from build123d import *

# Parameters (mm, degrees)
SKETCH1_W               = 15
SKETCH1_H               = 15
SKETCH1_R               = 2.5
BOSS_EXTRUDE1_DEPTH     = 90
SKETCH2_W               = 10.174
SKETCH2_H               = 10.174
CUT_EXTRUDE1_DEPTH      = 83
CUT_EXTRUDE2_DEPTH      = 83
CUT_EXTRUDE2_DEPTH_BACK = 83
SKETCH4_R               = 1.75
CUT_EXTRUDE3_DEPTH      = 83


with BuildPart() as part:
    # Sketch1 → Boss-Extrude1 (new body)
    with BuildSketch(Plane(origin=(0, 0, 0), x_dir=(1, 0, 0), z_dir=(0, 1, 0))):
        Rectangle(SKETCH1_W, SKETCH1_H)
        with Locations(Location((0, 0, 0), (0, 0, 270))):
            Circle(SKETCH1_R, mode=Mode.SUBTRACT)
    extrude(amount=-BOSS_EXTRUDE1_DEPTH)

    # Sketch2 → Cut-Extrude1 (cut)
    with BuildSketch(Plane(origin=(0, 0, 0), x_dir=(1, 0, 0), z_dir=(0, 1, 0))):
        Rectangle(SKETCH2_W, SKETCH2_H)
    extrude(amount=-CUT_EXTRUDE1_DEPTH, mode=Mode.SUBTRACT)

    # Sketch3 → Cut-Extrude2 (cut, two sides: drawn at the far end of the back side and taken through both)
    with BuildSketch(Plane(origin=(0, 0, 0), x_dir=(0, 0, -1), z_dir=(1, 0, 0)).offset(-CUT_EXTRUDE2_DEPTH_BACK)):
        Polygon((-7.5, 0), (7.5, -15), (7.5, 0), align=None)
    extrude(amount=CUT_EXTRUDE2_DEPTH + CUT_EXTRUDE2_DEPTH_BACK, mode=Mode.SUBTRACT)

    # Sketch4 → Cut-Extrude3 (cut)
    with BuildSketch(Plane.XY):
        with Locations((0, -10)):
            Circle(SKETCH4_R)
        with Locations((0, -20)):
            Circle(SKETCH4_R)
    extrude(amount=CUT_EXTRUDE3_DEPTH, mode=Mode.SUBTRACT)


solid = part.part
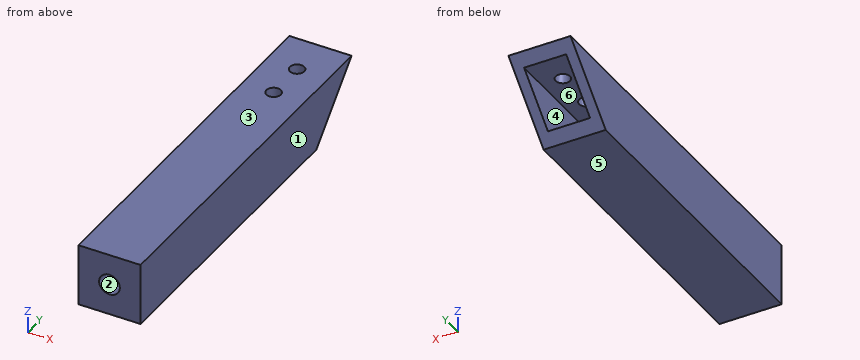
Source: CAD feature listing. Evaluate the final solid. Frame: model axes, mm. Face numbers are marked on the shaded views. A direction names the side the tool comes from. Round coordinates to 2 decimals unless told otherwise and drop trailing zeros. Loops run counter-clockwise (first coordinate to the right, second up) from the corner with the lowest first, then second, coordinate; pieces in that order, holes last. Notation, with made-up numbers: (54, 86.5) - (98, 86.5) arc R29 ccw to (98, 125.5) - close; hole circle Ø2 at (39.25, 21.5). An arc over 180 degrees is marked (long way). Write item = value, one per line. Start each with the question number.
Item 1: Section query A-A on z = 0. Output: boundary loops of the cut face in (x, y), plus the area to 3 significant figures.
Item 2: Mould query, pull axis Z, two halves, no side actions, for the marked faces 1, 2, 3 and 4. Classes: released by +Z, released by -Z, zero draft, split by the parting line, or undercut.
Item 3: Reachability of the marked faces 5 and 6 from +Z, -Z, +X, -X, +Y, -Y: full face, straight path, thin tool, end or side. Return the list, or none.
Item 4: First-contact query: pin 1 Ø5 at (x, z) = (2, -2) entering from +Y; pin 2 Ø5 at (x, z) = (6, 2) entering from +Y. Flat tips, straight axial feed; report the tip coordinate or a pass-through.
Item 5: Section query D-D on z = 4. Output: boundary loops of the cut face in (x, y).
Item 6: Material intervals for line 1 (Z direction, x = -2.5, y = -19); line 2 (X direction, y = -84.75, z = 0), sorted ascending.
Item 7: Section query B-B on x = 0. Output: boundary loops of the cut face in (y, z), plus the area to 3 significant figures.
Item 8: Section query C-C on y = -62. Output: boundary loops of the cut face in (x, z), plus the area to 3 significant figures.
Results list:
q1.outline = (-7.5, -90) - (-2.5, -90) - (-2.5, -83) - (-5.09, -83) - (-5.09, -7.5) - (-7.5, -7.5) - close; (2.5, -90) - (7.5, -90) - (7.5, -7.5) - (5.09, -7.5) - (5.09, -83) - (2.5, -83) - close
q1.area = 434 mm²
q2.face_1 = zero draft
q2.face_2 = undercut
q2.face_3 = released by +Z
q2.face_4 = undercut
q3.face_5 = -Z, +X, -X, +Y, -Y
q3.face_6 = +Y
q4.pin_1 = -83
q4.pin_2 = -3
q5.outline = (-7.5, -90) - (7.5, -90) - (7.5, -3.5) - (5.09, -3.5) - (5.09, -83) - (-5.09, -83) - (-5.09, -3.5) - (-7.5, -3.5) - close
q6.line_1 = -7.5 to -5.09, 5.09 to 7.5
q6.line_2 = -7.5 to -2.5, 2.5 to 7.5
q7.outline = (-90, -7.5) - (-15, -7.5) - (-12.59, -5.09) - (-83, -5.09) - (-83, -2.5) - (-90, -2.5) - close; (-90, 2.5) - (-83, 2.5) - (-83, 5.09) - (-21.75, 5.09) - (-21.75, 7.5) - (-90, 7.5) - close; (-18.25, 5.09) - (-11.75, 5.09) - (-11.75, 7.5) - (-18.25, 7.5) - close; (-8.25, 5.09) - (-2.41, 5.09) - (0, 7.5) - (-8.25, 7.5) - close
q7.area = 417 mm²
q8.outline = (-7.5, -7.5) - (7.5, -7.5) - (7.5, 7.5) - (-7.5, 7.5) - close; hole (-5.09, -5.09) - (5.09, -5.09) - (5.09, 5.09) - (-5.09, 5.09) - close
q8.area = 121 mm²
